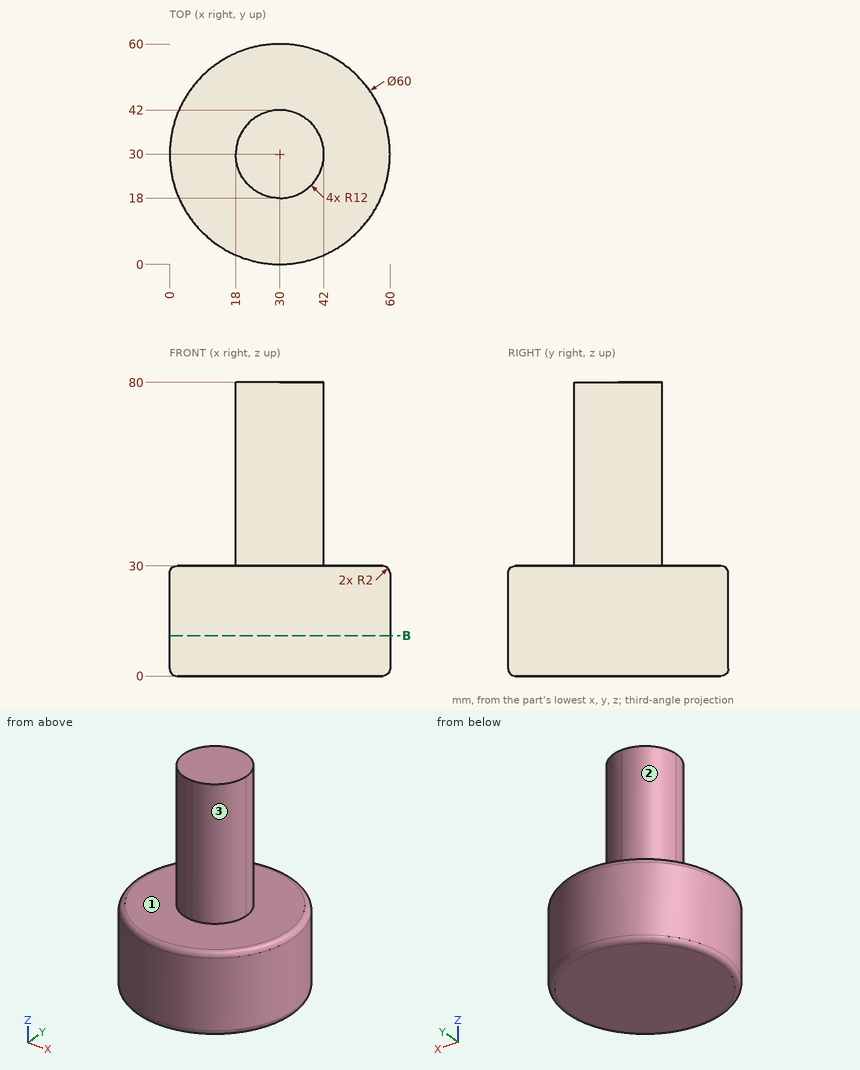
Design review of the part shown in the three views and the two pictorial views. Dimensions are in mm from the part's minimum x, y and z. A direction names the side the tool comes from. Round coordinates to 2 decimals unless told otherwise and drop trailing zeros. Write each loop counter-clockwise with the first axis right and the second up, starting at its lowest first coordinate (ties: lowest second). Pieces come first, ordered by that corner, then holes. Notation, with made-up numbers: M 41.5,29 L 55.5,29 A12 ccw 55.5,39 Z; hole C 28,52.25 d4. An arc over 180 degrees is marked long. One line per item, written item: value. Start each with the question number.
1. Clearance check with flat-ended pins moving along their axes: P1, Ø1.5, axis at y = 47, z = 29.5, coming from the -X side; P2, Ø1.5, axis at x = 46.5, y = 47.5, coming from the +Z side; P3, Ø2, axis at x = 40.5, z = 27, coming from the -Y side. State where each tip first meets the part, or that it passes through.
2. To check wall thickness, follow probe 1 along Z at (x, y) = (32.5, 12.5); probe 2 along Z at (x, y) = (47, 53.5); probe 3 along Y at (x, z) = (3, 28). State the ranges of each line that lie inside material, in increasing order. Write a range as from..to.
3. Take a section at B-B on z = 11. State the section outline as (x, y) points, then the cut area to 3 significant figures.
4. For the marked faces 1, 2 and 3, list the 3-axis set-ups (+Z, -Z, +X, -X, +Y, -Y) from which the entire face can be reached by the end or side of a thin tool; tool diameter is ignored.
Computed:
1. P1: stops at x = 5.23
1. P2: stops at z = 30
1. P3: stops at y = 1.54
2. probe 1: z = 0..30
2. probe 2: z = 0.27..29.73
2. probe 3: y = 16.92..43.08
3. outline: C 30,30 d60
3. area: 2,830 mm²
4. face 1: +Z
4. face 2: +Z, -X, +Y
4. face 3: +Z, +X, -Y
